```python
from build123d import *

# Parameters (mm, degrees)
F1_DEPTH = 6
F3_DEPTH = 3
F4_R     = 0.5
F5_DEPTH = 3
F6_SIZE  = 1


with BuildPart() as f1:
    # F0 (on Top) → F1 (new body)
    with BuildSketch(Plane.XY):
        Polygon((10, -5.35), (-10, -4.25), (-10.1647510023, -7.2454727686), (9.8352489977, -8.3454727686), align=None)
    extrude(amount=-F1_DEPTH)



with BuildPart() as f1b:
    # F0 (on Top) → F1, piece 2 (new body)
    with BuildSketch(Plane.XY):
        Polygon((9.8352489977, 8.3454727686), (-10.1647510023, 7.2454727686), (-10, 4.25), (10, 5.35), align=None)
    extrude(amount=-F1_DEPTH)


with BuildPart() as f1_1:
    add(f1.part)

    add(f1b.part)  # F3 merges F1b
    # F2 (on face) → F3 (join)
    with BuildSketch(Plane.XY):
        Polygon((10, 5.35), (-10, 4.25), (-10, -4.25), (10, -5.35), align=None)
    extrude(amount=-F3_DEPTH)

    # F4 (on face) → F5 (cut)
    with BuildSketch(Plane.XY):
        with Locations((-7.5, 0)):
            Circle(F4_R)
        with Locations((7.5, 0)):
            Circle(F4_R)
    extrude(amount=-F5_DEPTH, mode=Mode.SUBTRACT)

    # F6
    f6_edges = [f1_1.edges().sort_by_distance(p)[0] for p in [
        (-10, 4.25, -4.5),
        (-10, 4.25, -1.5),
        (10, 5.35, -1.5),
        (10, 5.35, -4.5),
        (10, -5.35, -1.5),
        (10, -5.35, -4.5),
        (-10, -4.25, -4.5),
        (-10, -4.25, -1.5),
    ]]
    chamfer(f6_edges, length=F6_SIZE)


solid = f1_1.part
```
For this review, take the finished solid that the model builds, in its own axes (mm). A direction names the side the tool comes from. Round coordinates to 2 decimals unless told otherwise and drop trailing zeros. Loops run counter-clockwise (first coordinate to the right, second up) from the corner with the lowest first, then second, coordinate; pieces in that order, holes last.
Q1. To check wall thickness, follow line 1 along Z through (x, y) = (-1, -3); line 2 along Y through (x, z) = (-7.5, -1.3); line 3 along Y through (x, z) = (-1, -3.4) (3 decimals). State the ranges of each line that lie inside material, in increasing order.
Result sheet:
line 1: z = -3 to 0
line 2: y = -7.39 to -0.5, 0.5 to 7.39
line 3: y = -7.75 to -4.745, 4.745 to 7.75
Q2. Insertion check: pin 1 Ø2.5 at (y, z) = (0, -1.5) entering from -X; pin 2 Ø4 at (x, y) = (3, 1) entering from -Z. Each pin has a flat end and moves straight along its axis. Give the tip position at first contact, or say it passes through.
Result sheet:
pin 1: stops at x = -10
pin 2: stops at z = -3
Q3. Add section B-B on x = -7.25. Write out the cut boundary in (y, z).
Result sheet:
outline: (-7.41, -6) - (-4.4, -6) - (-4.4, -3) - (-0.43, -3) - (-0.43, 0) - (-7.41, 0) - close; (0.43, -3) - (4.4, -3) - (4.4, -6) - (7.41, -6) - (7.41, 0) - (0.43, 0) - close
Q4. Add section D-D on z = -1.1. Write out the cut boundary in (x, y), plus the area to 3 significant figures.
Result sheet:
outline: (-10.16, -7.25) - (9.84, -8.35) - (10, -5.35) - (10, 5.35) - (9.84, 8.35) - (-10.16, 7.25) - (-10, 4.25) - (-10, -4.25) - close; hole circle Ø1 at (-7.5, 0); hole circle Ø1 at (7.5, 0)
area: 311 mm2
Q5. Machinability: for faces 1 (the face through (0.126, -4.807, -4.479)), 2 (the face through (-9.52, -4.77, -4.48)), 3 (the face through (-10.1, 6.1, -3)), which of the approach directions +Z, -Z, +X, -X, +Y, -Y give a long, thin tool a straight path to every point of the face, cutting with its end or side? Answer none if there is none.
Result sheet:
face 1: -Z, +X
face 2: -Z, -X
face 3: +Z, -Z, -X
Q6. Mouldability with a two-part tool opening along X and no side actions: class faces 4 (the face through (8, 0, -1)), 5 (the face through (10, 0, -1)), 6 (the face through (0, 0, -3)), 7 (the face through (-7, 0, -1)) as +X half, -X half, draft (parallel to the pull), parting line (faces both ways), or undercut.
Result sheet:
face 4: undercut
face 5: +X half
face 6: draft
face 7: undercut
Q7. Add section A-A on y = 0. Write out the cut boundary in (x, z), plus the area to 3 significant figures.
Result sheet:
outline: (-10, -3) - (-8, -3) - (-8, 0) - (-10, 0) - close; (-7, -3) - (7, -3) - (7, 0) - (-7, 0) - close; (8, -3) - (10, -3) - (10, 0) - (8, 0) - close
area: 54.0 mm2
Q8. Add section C-C on z = -4.2. Write out the cut boundary in (x, y).
Result sheet:
outline: (-10.16, -7.25) - (9.84, -8.35) - (9.95, -6.35) - (9, -5.3) - (-9, -4.3) - (-10.05, -5.25) - close; (-10.16, 7.25) - (-10.05, 5.25) - (-9, 4.3) - (9, 5.3) - (9.95, 6.35) - (9.84, 8.35) - close
